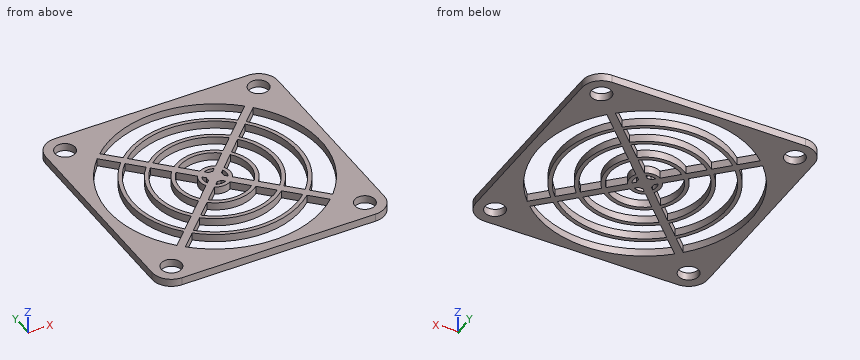
from build123d import *

# Parameters (mm, degrees)
F0_W     = 60
F0_H     = 60
F0_R     = 2.6
F1_DEPTH = 2
F2_R     = 5


with BuildPart() as f1:
    # F0 (on Top) → F1 (new body)
    with BuildSketch(Plane.XY):
        Rectangle(F0_W, F0_H)
        with Locations((-25, -25)):
            Circle(F0_R, mode=Mode.SUBTRACT)
        with BuildLine():
            Line((-15.539504, 14.12529), (-11.998697, 10.584483))
            ThreePointArc((-11.998697, 10.584483), (-16, 0), (-11.998697, -10.584483))
            Line((-11.998697, -10.584483), (-15.539504, -14.12529))
            ThreePointArc((-15.539504, -14.12529), (-21, 0), (-15.539504, 14.12529))
        make_face(mode=Mode.SUBTRACT)
        with BuildLine():
            ThreePointArc((18.725469, -20.139683), (0, -27.5), (-18.725469, -20.139683))
            Line((-18.725469, -20.139683), (-14.833163, -16.247377))
            ThreePointArc((-14.833163, -16.247377), (0, -22), (14.833163, -16.247377))
            Line((14.833163, -16.247377), (18.725469, -20.139683))
        make_face(mode=Mode.SUBTRACT)
        with BuildLine():
            ThreePointArc((14.12529, -15.539504), (0, -21), (-14.12529, -15.539504))
            Line((-14.12529, -15.539504), (-10.584483, -11.998697))
            ThreePointArc((-10.584483, -11.998697), (0, -16), (10.584483, -11.998697))
            Line((10.584483, -11.998697), (14.12529, -15.539504))
        make_face(mode=Mode.SUBTRACT)
        with Locations((25, -25)):
            Circle(F0_R, mode=Mode.SUBTRACT)
        with BuildLine():
            Line((-9.875898, -11.290112), (-6.328517, -7.74273))
            ThreePointArc((-6.328517, -7.74273), (0, -10), (6.328517, -7.74273))
            Line((6.328517, -7.74273), (9.875898, -11.290112))
            ThreePointArc((9.875898, -11.290112), (0, -15), (-9.875898, -11.290112))
        make_face(mode=Mode.SUBTRACT)
        with BuildLine():
            Line((-5.617449, -7.031662), (-2.031506, -3.44572))
            ThreePointArc((-2.031506, -3.44572), (0, -4), (2.031506, -3.44572))
            Line((2.031506, -3.44572), (5.617449, -7.031662))
            ThreePointArc((5.617449, -7.031662), (0, -9), (-5.617449, -7.031662))
        make_face(mode=Mode.SUBTRACT)
        with BuildLine():
            Line((0.517638, -1.931852), (1.292893, -2.707107))
            ThreePointArc((1.292893, -2.707107), (0, -3), (-1.292893, -2.707107))
            Line((-1.292893, -2.707107), (-0.517638, -1.931852))
            ThreePointArc((-0.517638, -1.931852), (0, -2), (0.517638, -1.931852))
        make_face(mode=Mode.SUBTRACT)
        with BuildLine():
            Line((-20.139683, 18.725469), (-16.247377, 14.833163))
            ThreePointArc((-16.247377, 14.833163), (-22, 0), (-16.247377, -14.833163))
            Line((-16.247377, -14.833163), (-20.139683, -18.725469))
            ThreePointArc((-20.139683, -18.725469), (-27.5, 0), (-20.139683, 18.725469))
        make_face(mode=Mode.SUBTRACT)
        with BuildLine():
            ThreePointArc((-11.290112, -9.875898), (-15, 0), (-11.290112, 9.875898))
            Line((-11.290112, 9.875898), (-7.74273, 6.328517))
            ThreePointArc((-7.74273, 6.328517), (-10, 0), (-7.74273, -6.328517))
            Line((-7.74273, -6.328517), (-11.290112, -9.875898))
        make_face(mode=Mode.SUBTRACT)
        with BuildLine():
            ThreePointArc((-7.031662, -5.617449), (-9, 0), (-7.031662, 5.617449))
            Line((-7.031662, 5.617449), (-3.44572, 2.031506))
            ThreePointArc((-3.44572, 2.031506), (-4, 0), (-3.44572, -2.031506))
            Line((-3.44572, -2.031506), (-7.031662, -5.617449))
        make_face(mode=Mode.SUBTRACT)
        with BuildLine():
            ThreePointArc((-2.707107, -1.292893), (-3, 0), (-2.707107, 1.292893))
            Line((-2.707107, 1.292893), (-1.931852, 0.517638))
            ThreePointArc((-1.931852, 0.517638), (-2, 0), (-1.931852, -0.517638))
            Line((-1.931852, -0.517638), (-2.707107, -1.292893))
        make_face(mode=Mode.SUBTRACT)
        with Locations((-25, 25)):
            Circle(F0_R, mode=Mode.SUBTRACT)
        with BuildLine():
            Line((2.707107, -1.292893), (1.931852, -0.517638))
            ThreePointArc((1.931852, -0.517638), (2, 0), (1.931852, 0.517638))
            Line((1.931852, 0.517638), (2.707107, 1.292893))
            ThreePointArc((2.707107, 1.292893), (3, 0), (2.707107, -1.292893))
        make_face(mode=Mode.SUBTRACT)
        with BuildLine():
            Line((-0.517638, 1.931852), (-1.292893, 2.707107))
            ThreePointArc((-1.292893, 2.707107), (0, 3), (1.292893, 2.707107))
            Line((1.292893, 2.707107), (0.517638, 1.931852))
            ThreePointArc((0.517638, 1.931852), (0, 2), (-0.517638, 1.931852))
        make_face(mode=Mode.SUBTRACT)
        with BuildLine():
            Line((7.031662, -5.617449), (3.44572, -2.031506))
            ThreePointArc((3.44572, -2.031506), (4, 0), (3.44572, 2.031506))
            Line((3.44572, 2.031506), (7.031662, 5.617449))
            ThreePointArc((7.031662, 5.617449), (9, 0), (7.031662, -5.617449))
        make_face(mode=Mode.SUBTRACT)
        with BuildLine():
            Line((-2.031506, 3.44572), (-5.617449, 7.031662))
            ThreePointArc((-5.617449, 7.031662), (0, 9), (5.617449, 7.031662))
            Line((5.617449, 7.031662), (2.031506, 3.44572))
            ThreePointArc((2.031506, 3.44572), (0, 4), (-2.031506, 3.44572))
        make_face(mode=Mode.SUBTRACT)
        with BuildLine():
            ThreePointArc((11.290112, 9.875898), (15, 0), (11.290112, -9.875898))
            Line((11.290112, -9.875898), (7.74273, -6.328517))
            ThreePointArc((7.74273, -6.328517), (10, 0), (7.74273, 6.328517))
            Line((7.74273, 6.328517), (11.290112, 9.875898))
        make_face(mode=Mode.SUBTRACT)
        with BuildLine():
            Line((-6.328517, 7.74273), (-9.875898, 11.290112))
            ThreePointArc((-9.875898, 11.290112), (0, 15), (9.875898, 11.290112))
            Line((9.875898, 11.290112), (6.328517, 7.74273))
            ThreePointArc((6.328517, 7.74273), (0, 10), (-6.328517, 7.74273))
        make_face(mode=Mode.SUBTRACT)
        with BuildLine():
            Line((15.539504, -14.12529), (11.998697, -10.584483))
            ThreePointArc((11.998697, -10.584483), (16, 0), (11.998697, 10.584483))
            Line((11.998697, 10.584483), (15.539504, 14.12529))
            ThreePointArc((15.539504, 14.12529), (21, 0), (15.539504, -14.12529))
        make_face(mode=Mode.SUBTRACT)
        with BuildLine():
            Line((16.247377, 14.833163), (20.139683, 18.725469))
            ThreePointArc((20.139683, 18.725469), (27.5, 0), (20.139683, -18.725469))
            Line((20.139683, -18.725469), (16.247377, -14.833163))
            ThreePointArc((16.247377, -14.833163), (22, 0), (16.247377, 14.833163))
        make_face(mode=Mode.SUBTRACT)
        with BuildLine():
            Line((-10.584483, 11.998697), (-14.12529, 15.539504))
            ThreePointArc((-14.12529, 15.539504), (0, 21), (14.12529, 15.539504))
            Line((14.12529, 15.539504), (10.584483, 11.998697))
            ThreePointArc((10.584483, 11.998697), (0, 16), (-10.584483, 11.998697))
        make_face(mode=Mode.SUBTRACT)
        with BuildLine():
            Line((-14.833163, 16.247377), (-18.725469, 20.139683))
            ThreePointArc((-18.725469, 20.139683), (0, 27.5), (18.725469, 20.139683))
            Line((18.725469, 20.139683), (14.833163, 16.247377))
            ThreePointArc((14.833163, 16.247377), (0, 22), (-14.833163, 16.247377))
        make_face(mode=Mode.SUBTRACT)
        with Locations((25, 25)):
            Circle(F0_R, mode=Mode.SUBTRACT)
    extrude(amount=F1_DEPTH)

    # F2
    f2_edges = [f1.edges().sort_by_distance(p)[0] for p in [
        (30, 30, 1),
        (-30, 30, 1),
        (-30, -30, 1),
        (30, -30, 1),
    ]]
    fillet(f2_edges, radius=F2_R)


solid = f1.part
Input: part model. Units: mm. Frame: model coordinates. Give positions to 0.01 mm unless a question says otherwise; leave off trailing zeros. Order: outer loops, then holes, each group sorted by start corner. A loop starts at its lowest first (then second) coordinate and runs counter-clockwise, first axis right, second up. Notation, with made-up numbers: (0, 64.25) -> (27, 64.25) arc R36 ccw to (27, 100.25) -> close; hole circle Ø10 at (65.5, 74). An arc over 180 degrees is marked (long way). Use one line per item in the form item = value.
1) Line query: probe 1 along Y at (x, z) = (-25, 0.7); probe 2 along X at (y, z) = (-11, 1.7); probe 3 along Y at (x, z) = (18.5, 0.7). Output: solid intervals per line, ascending.
Response values:
probe_1 = -30 to -27.6, -22.4 to -11.46, 11.46 to 22.4, 27.6 to 30
probe_2 = -30 to -25.2, -19.05 to -17.89, -12.41 to -9.59, 9.59 to 12.41, 17.89 to 19.05, 25.2 to 30
probe_3 = -30 to -20.35, -19.91 to -17.09, -11.91 to -9.94, 9.94 to 11.91, 17.09 to 19.91, 20.35 to 30
2) Section B-B, the plane z = 0.6. Count the separate pieces of the cut face and the enclosed holes in it, and give its area (3 significant figures).
Response values:
separate_pieces = 1
enclosed_holes = 24
area = 1,620 mm^2
3) Section A-A, the plane x = -23.5. Return loops of the section in (y, z), and give its area (3 significant figures).
Response values:
outline = (-30, 0) -> (-27.12, 0) -> (-27.12, 2) -> (-30, 2) -> close; (-22.88, 0) -> (-14.28, 0) -> (-14.28, 2) -> (-22.88, 2) -> close; (14.28, 0) -> (22.88, 0) -> (22.88, 2) -> (14.28, 2) -> close; (27.12, 0) -> (30, 0) -> (30, 2) -> (27.12, 2) -> close
area = 45.9 mm^2
